Verification items for the finished model (mm, model axes). A direction names the side the tool comes from. Round coordinates to 2 decimals unless told otherwise and drop trailing zeros. Loops run counter-clockwise (first coordinate to the right, second up) from the corner with the lowest first, then second, coordinate; pieces in that order, holes last. Notation, with made-up numbers: (63, 53.25) - (120, 53.25) arc R34 cw to (120, 91.25) - close; hole circle Ø7 at (0, -40). An arc over 180 degrees is marked (long way). Use a Markdown table: item, result. Add a question column.
```python
from build123d import *

# Parameters (mm, degrees)
SKETCH1_W           = 108.2
SKETCH1_H           = 50
BOSS_EXTRUDE1_DEPTH = 6
SKETCH2_W           = 50
SKETCH2_H           = 6
BOSS_EXTRUDE2_DEPTH = 6
SKETCH3_W           = 50
SKETCH3_H           = 6
BOSS_EXTRUDE3_DEPTH = 6
SKETCH4_W           = 108.2
SKETCH4_H           = 6
BOSS_EXTRUDE4_DEPTH = 10
SKETCH5_W           = 108.2
SKETCH5_H           = 6
BOSS_EXTRUDE5_DEPTH = 10


with BuildPart() as part:
    # Sketch1 → Boss-Extrude1 (new body)
    with BuildSketch(Plane(origin=(0, 0, 0), x_dir=(1, 0, 0), z_dir=(0, 1, 0))):
        with Locations((54.1, 25)):
            Rectangle(SKETCH1_W, SKETCH1_H)
    extrude(amount=BOSS_EXTRUDE1_DEPTH)

    # Sketch2 → Boss-Extrude2 (add)
    with BuildSketch(Plane.ZY):
        with Locations((-25, 3)):
            Rectangle(SKETCH2_W, SKETCH2_H)
    extrude(amount=BOSS_EXTRUDE2_DEPTH)

    # Sketch3 → Boss-Extrude3 (add)
    with BuildSketch(Plane(origin=(108.2, 0, 0), x_dir=(0, 0, -1), z_dir=(1, 0, 0))):
        with Locations((25, 3)):
            Rectangle(SKETCH3_W, SKETCH3_H)
    extrude(amount=BOSS_EXTRUDE3_DEPTH)

    # Sketch4 → Boss-Extrude4 (add)
    with BuildSketch(Plane(origin=(0, 0, -50), x_dir=(-1, 0, 0), z_dir=(0, 0, -1))):
        with Locations((-54.1, 3)):
            Rectangle(SKETCH4_W, SKETCH4_H)
    extrude(amount=BOSS_EXTRUDE4_DEPTH)

    # Sketch5 → Boss-Extrude5 (add)
    with BuildSketch(Plane.XY):
        with Locations((54.1, 3)):
            Rectangle(SKETCH5_W, SKETCH5_H)
    extrude(amount=BOSS_EXTRUDE5_DEPTH)


solid = part.part
```
Q1. Thickness scan on line 1 along X through (y, z) = (1.15, -51.5). Record the ranges inside material, lowest first.
Q2. Section check B-B on z = 4.5. Record the cut outline in (x, y), plus the area to 3 significant figures.
Q3. Section check A-A on y = 2.55. Record the cut outline in (x, z), plus the area to 3 significant figures.
Q4. Go/stop test with flat-tipped pins: pin 1 Ø3 at (y, z) = (4, 7) entering from -X; pin 2 Ø1.8 at (x, y) = (-1.5, 3) entering from -Z; pin 3 Ø1.8 at (x, y) = (-2, 3.5) entering from +Z; pin 4 Ø5 at (x, z) = (98.5, -49) entering from -Y. Record where each tip stops, or that it passes through.
Q5. Set-up check for faces 1 (the face through (-3, 3, -50)), 2 (the face through (0, 3, 5)), 3 (the face through (108.2, 3, 5)), 4 (the face through (108.2, 3, -55)): record each of +Z, -Z, +X, -X, +Y, -Y from which the full face is reachable in a straight line by a thin tool's end or side.
Determined:
| question | item | result |
|---|---|---|
| 1 | line 1 | x = 0 to 108.2 |
| 2 | outline | (0, 0) - (108.2, 0) - (108.2, 6) - (0, 6) - close |
| 2 | area | 649 mm² |
| 3 | outline | (-6, -50) - (0, -50) - (0, -60) - (108.2, -60) - (108.2, -50) - (114.2, -50) - (114.2, 0) - (108.2, 0) - (108.2, 10) - (0, 10) - (0, 0) - (-6, 0) - close |
| 3 | area | 8,170 mm² |
| 4 | pin 1 | stops at x = 0 |
| 4 | pin 2 | stops at z = -50 |
| 4 | pin 3 | stops at z = 0 |
| 4 | pin 4 | stops at y = 0 |
| 5 | face 1 | -Z, -X, +Y, -Y |
| 5 | face 2 | +Z, -X, +Y, -Y |
| 5 | face 3 | +Z, +X, +Y, -Y |
| 5 | face 4 | -Z, +X, +Y, -Y |
